Autodesk Inventor part; units mm, degrees
ref_plane "YZ Plane" through (0, 0, 0) normal (1, 0, 0) x (0, 1, 0)
ref_plane "XZ Plane" through (0, 0, 0) normal (0, 1, 0) x (-1, 0, 0)
ref_plane "XY Plane" through (0, 0, 0) normal (0, 0, 1) x (1, 0, 0)
sketch "Sketch1" plane through (0, 0, 0) normal (0, 1, 0) x (-1, 0, 0)
  line L0 (28.75, 45) -> (-28.75, 45) construction
  line L1 (-28.75, 45) -> (-28.75, -41.6)
  line L2 (-28.75, -41.6) -> (28.75, -41.6)
  line L3 (28.75, -41.6) -> (28.75, 45)
  line L4 (28.75, 45) -> (-28.75, -41.6) construction
  line L5 (-28.75, 45) -> (28.75, -41.6) construction
  line L6 (45, 45) -> (-45, 45)
  line L7 (-45, 45) -> (-45, -45)
  line L8 (-45, -45) -> (45, -45)
  line L9 (45, -45) -> (45, 45)
  line L10 (45, 45) -> (-45, -45) construction
  line L11 (-45, 45) -> (45, -45) construction
  point P0 (0, 0)
  point P1 (0, 1.7)
  point P2 (28.75, 45)
  dimension "d0" = 57.5
  dimension "d1" = 86.6
  dimension "d2" = 90
  dimension "d3" = 90
  dimension "d4" = 0
  dimension "d5" = 0
extrude "Extrusion1" add sketch "Sketch1" against normal blind 3
extrude "Extrusion2" add sketch "Sketch1" along normal blind 17 contours L1 L2 L3 L6 L9 L8 L7
chamfer "Chamfer1" distance 10 angle 45 4 edges at (-45, 7, 45) (-45, 7, -45) (45, 7, -45) (45, 7, 45)
sketch "Sketch2" plane through (-45, -3, -35) normal (-1, 0, 0) x (0, 0, 1)
  line L0 (-6.6, 3) -> (-6.6, 20)
  line L1 (-6.6, 3) -> (8.4, 3)
  line L2 (8.4, 3) -> (8.4, 8)
  line L3 (8.4, 8) -> (-6.6, 8)
  line L4 (-6.6, 8) -> (-6.6, 3)
  point P0 (35, 3)
  dimension "d13" = 15
  dimension "d14" = 5
extrude "Extrusion3" cut sketch "Sketch2" against normal blind 16.75
properties part number "console case"
Read the model definition and answer for the solid it produces. Units are mm, in the model's axes. A direction names the side the tool comes from. Round coordinates to 2 decimals unless told otherwise and drop trailing zeros. Write each loop counter-clockwise with the first axis right and the second up, starting at its lowest first coordinate (ties: lowest second). Pieces come first, ordered by that corner, then holes.
1. Given pin 1 Ø2 at (x, y) = (8, 12) entering from +Z; pin 2 Ø3 at (x, z) = (-10.5, 26.5) entering from +Y; pin 3 Ø1.5 at (x, y) = (-41, 1.5) entering from -Z, each flat-ended and moving along its own axis, determine where each tip first touches the part or whether it passes through.
2. Determine the mould class of faces 1 (the face through (-37, 2, -26.6)), 2 (the face through (-40, 7, 40)), 3 (the face through (-45, 7, 0)) for opening direction Z: pulls with the +Z half, pulls with the -Z half, needs draft (parallel to the pull), parting line crosses it, or undercut.
3. The part is cut by section B-B, the plane z = -31.5. Determine the outline of the cut face in (x, y).
4. Which of the six approach directions +Z, -Z, +X, -X, +Y, -Y give full straight-line access (tool end or side, diameter ignored) to faces 4 (the face through (-40, 9, -40)), 5 (the face through (-28.75, 8, 1)), 6 (the face through (-37, 5, -34))?
5. The part is cut by section A-A, the plane y = 3. Determine the outline of the cut face in (x, z), then the cut area to 3 significant figures.
6. Straight lines are drawn through the part: L1, parallel to X at y = 9.5, z = -27; L2, parallel to Z at x = 26, y = 10; L3, parallel to Y at x = -12, z = 38. For each, find the intervals that lie inside material, in ascending order.
7. The part is cut by section C-C, the plane x = -31. Determine the outline of the cut face in (y, z).
8. The part is cut by section D-D, the plane z = -22. Determine the outline of the cut face in (x, y), then the cut area to 4 significant figures.
Values:
1. pin 1: stops at z = -41.6
1. pin 2: stops at y = 0
1. pin 3: stops at z = -26.6
2. face 1: undercut
2. face 2: pulls with the +Z half
2. face 3: needs draft
3. outline: (-45, -3) - (45, -3) - (45, 17) - (28.75, 17) - (28.75, 0) - (-45, 0) - close; (-45, 5) - (-28.75, 5) - (-28.75, 17) - (-45, 17) - close
4. face 4: -Z, -X, +Y, -Y
4. face 5: +Z, +Y
4. face 6: -X
5. outline: (-45, -26.6) - (-28.75, -26.6) - (-28.75, 45) - (-35, 45) - (-45, 35) - close; (-38.4, -41.6) - (-35, -45) - (35, -45) - (45, -35) - (45, 35) - (35, 45) - (28.75, 45) - (28.75, -41.6) - close
5. area: 2,700 mm2
6. L1: x = -45 to -28.75, 28.75 to 45
6. L2: z = -45 to -41.6
6. L3: y = -3 to 0
7. outline: (-3, -45) - (17, -45) - (17, 45) - (-3, 45) - close; hole (0, -41.6) - (5, -41.6) - (5, -26.6) - (0, -26.6) - close
8. outline: (-45, -3) - (45, -3) - (45, 17) - (28.75, 17) - (28.75, 0) - (-28.75, 0) - (-28.75, 17) - (-45, 17) - close
8. area: 822.5 mm2
